Autodesk Inventor part; units mm, degrees
ref_plane "YZ Plane" through (0, 0, 0) normal (1, 0, 0) x (0, 1, 0)
ref_plane "XZ Plane" through (0, 0, 0) normal (0, 1, 0) x (-1, 0, 0)
ref_plane "XY Plane" through (0, 0, 0) normal (0, 0, 1) x (1, 0, 0)
sketch "スケッチ1" plane through (0, 0, 0) normal (0, 0, 1) x (1, 0, 0)
  line L0 (-27.5, -75) -> (27.5, -75)
  line L1 (27.5, -75) -> (27.5, 75)
  line L2 (27.5, 75) -> (-27.5, 75)
  line L3 (-27.5, 75) -> (-27.5, -75)
  line L4 (-27.5, -75) -> (27.5, 75) construction
  line L5 (27.5, -75) -> (-27.5, 75) construction
  point P0 (0, 0)
  dimension "d0" = 55
  dimension "d1" = 150
extrude "押し出し1" add sketch "スケッチ1" along normal blind 5
sketch "スケッチ2" plane through (0, 0, 5) normal (0, 0, 1) x (1, 0, 0)
  line L0 (27.5, 75) -> (-27.5, 75)
  line L1 (-8.5, -75) -> (8.5, -75)
  line L2 (8.5, -75) -> (8.5, 75)
  line L3 (8.5, 75) -> (-8.5, 75)
  line L4 (-8.5, 75) -> (-8.5, -75)
  line L5 (-8.5, -75) -> (8.5, 75) construction
  line L6 (8.5, -75) -> (-8.5, 75) construction
  point P0 (0, 0)
  dimension "d4" = 17
extrude "押し出し2" add sketch "スケッチ2" along normal blind 8
sketch "スケッチ3" plane through (-27.5, 75, 0) normal (0, 1, 0) x (1, 0, 0)
  line L0 (55, 0) -> (0, 0)
  line L1 (0, 0) -> (0, -5)
  line L2 (19, -5) -> (0, -5)
  line L3 (19, -5) -> (19, -13)
  line L4 (36, -13) -> (19, -13)
  line L5 (36, -5) -> (36, -13)
  line L6 (55, -5) -> (36, -5)
  line L7 (55, 0) -> (55, -5)
  line L8 (36, -5) -> (36, -13)
  line L9 (19, -5) -> (36, -5)
  line L10 (36, -5) -> (36, -10)
  line L11 (36, -10) -> (19, -10)
  line L12 (19, -10) -> (19, -5)
  line L13 (22, -5) -> (33, -5)
  line L14 (33, -5) -> (33, -10)
  line L15 (33, -10) -> (22, -10)
  line L16 (22, -10) -> (22, -5)
  line L17 (19, -13) -> (36, -13)
  line L18 (24.5, -10) -> (30.5, -10)
  line L19 (30.5, -10) -> (30.5, -13)
  line L20 (30.5, -13) -> (24.5, -13)
  line L21 (24.5, -13) -> (24.5, -10)
  line L22 (24.5, -5) -> (30.5, -5)
  line L23 (30.5, -5) -> (30.5, -3)
  line L24 (30.5, -3) -> (24.5, -3)
  line L25 (24.5, -3) -> (24.5, -5)
  point P0 (27.5, 0)
  dimension "d7" = 5
  dimension "d8" = 11
  dimension "d9" = 3
  dimension "d10" = 6
  dimension "d11" = 5.5
  dimension "d14" = 2
extrude "押し出し3" cut sketch "スケッチ3" against normal through all contours L14 L11 L16 L9 | L9 L25 L24 L23 | L4 L21 L11 L19
sketch "スケッチ4" plane through (0, 0, 0) normal (0, 0, -1) x (-1, 0, 0)
  line L0 (27.5, -75) -> (-27.5, -75)
  line L1 (-27.5, -75) -> (-27.5, 75)
  point P0 (0, 0)
  point P1 (-22.5, -65)
  point P2 (22.5, -65)
  dimension "d15" = 10
  dimension "d16" = 10
  dimension "d17" = 45
  dimension "d18" = 5
hole "穴1" at (22.5, -65, 0) at (-22.5, -65, 0) direction (0, 0, 1) diameter 2.5 end through all
fillet "フィレット1" radius 2 8 edges at (-8.5, 0, 5) (8.5, 0, 5) (8.5, 0, 13) (-8.5, 0, 13) (27.5, -75, 2.5) (-27.5, -75, 2.5) (27.5, 75, 2.5) (-27.5, 75, 2.5)
properties part number "slide_part"
Design review of the part built by this model. Coordinates are the model's own, in mm. A direction names the side the tool comes from. Coordinates: 2 decimals unless noted, no trailing zeros. Loops run counter-clockwise (first coordinate to the right, second up) from the corner with the lowest first, then second, coordinate; pieces in that order, holes last.
Q1. We need section A-A on y = 28.5. State the section outline as (x, z) points, and give its area (3 significant figures).
Reported:
outline: (-27.5, 0) - (27.5, 0) - (27.5, 5) - (10.5, 5) arc R2 cw to (8.5, 7) - (8.5, 11) arc R2 ccw to (6.5, 13) - (3, 13) - (3, 10) - (5.5, 10) - (5.5, 5) - (3, 5) - (3, 3) - (-3, 3) - (-3, 5) - (-5.5, 5) - (-5.5, 10) - (-3, 10) - (-3, 13) - (-6.5, 13) arc R2 ccw to (-8.5, 11) - (-8.5, 7) arc R2 cw to (-10.5, 5) - (-27.5, 5) - close
area: 326 mm2
Q2. For pin 1 (5 mm diameter, centred on x = -1, y = 12, fed in from +Z); pin 2 (18.5 mm diameter, centred on x = 21, y = 30.5, fed in from +Z); pin 3 (2.5 mm diameter, centred on y = 5, z = 7, fed in from +X); pin 4 (2.5 mm diameter, centred on y = 25.5, z = 12, fed in from +X), all flat-tipped, find the tip position at first contact; note any pin that passes through.
Reported:
pin 1: stops at z = 13
pin 2: stops at z = 5
pin 3: stops at x = 8.94
pin 4: stops at x = 8.5
Q3. The part is to be moulded in two halves that separate along Y. For faces 4 (the face through (0, 75, 2)), 5 (the face through (22.12, -63.81, 2.54)), 6 (the face through (-3, 1, 12)), 7 (the face through (0, -75, 2)), say which applies: +Y half, -Y half, draft (parallel to the pull), parting line (faces both ways), or undercut.
Reported:
face 4: +Y half
face 5: undercut
face 6: draft
face 7: -Y half
Q4. To check wall thickness, follow line 1 (X direction, y = -65, z = 1.7); line 2 (X direction, y = -45, z = 10.5); line 3 (X direction, y = -45, z = 4.75). State the ranges of each line that lie inside material, in increasing order.
Reported:
line 1: x = -27.5 to -23.75, -21.25 to 21.25, 23.75 to 27.5
line 2: x = -8.5 to -3, 3 to 8.5
line 3: x = -27.5 to -3, 3 to 27.5
Q5. Tool access review of faces 1 (the face through (-4, 1, 5)), 2 (the face through (3, 1, 11)), 3 (the face through (-8.5, 1, 9)): name each direction out of +Z, -Z, +X, -X, +Y, -Y from which nothing blocks a thin tool from reaching the whole face with its end or side.
Reported:
face 1: +Y, -Y
face 2: +Z, +Y, -Y
face 3: +Z, -X, +Y, -Y
